from build123d import *

# Parameters (mm, degrees)
SKETCH1_W           = 5
SKETCH1_H           = 30
SKETCH1_R           = 1.55
BOSS_EXTRUDE1_DEPTH = 3
FILLET1_R           = 2.5


with BuildPart() as part:
    # Sketch1 → Boss-Extrude1 (new body)
    with BuildSketch(Plane(origin=(0, 0, 0), x_dir=(1, 0, 0), z_dir=(0, 1, 0))):
        Rectangle(SKETCH1_W, SKETCH1_H)
        with Locations(Location((0, 12, 0), (0, 0, 270))):
            Circle(SKETCH1_R, mode=Mode.SUBTRACT)
        with Locations(Location((0, -12, 0), (0, 0, 270))):
            Circle(SKETCH1_R, mode=Mode.SUBTRACT)
    extrude(amount=BOSS_EXTRUDE1_DEPTH)

    # Fillet1
    fillet1_edges = [part.edges().sort_by_distance(p)[0] for p in [
        (-2.5, 1.5, 15),
        (-2.5, 1.5, -15),
        (2.5, 1.5, -15),
        (2.5, 1.5, 15),
    ]]
    fillet(fillet1_edges, radius=FILLET1_R - 0.0001)  # a hair under: the kernel refuses the full size


solid = part.part
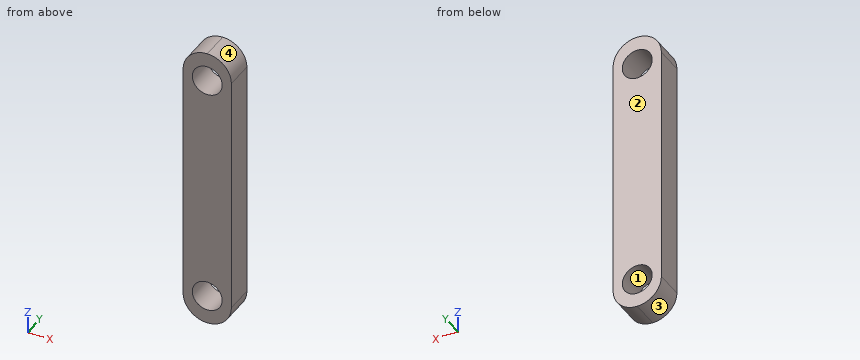
Build history of the part. All positions in model axes, mm. Face numbers are marked on the shaded views. Round coordinates to 2 decimals unless told otherwise and drop trailing zeros. Write each loop counter-clockwise with the first axis right and the second up, starting at its lowest first coordinate (ties: lowest second). Pieces come first, ordered by that corner, then holes. Notation, with made-up numbers: (62.5, -10) -> (121.5, -10) arc R10 cw to (121.5, 6) -> close; hole circle Ø11 at (78.25, 76). An arc over 180 degrees is marked (long way). Use one line per item in the form item = value.
Q1. Band-saw the part on A-A, the plane z = 12. Write the cut outline in (x, y).
Conclusion:
outline = (-2.5, 0) -> (-1.55, 0) -> (-1.55, 3) -> (-2.5, 3) -> close; (1.55, 0) -> (2.5, 0) -> (2.5, 3) -> (1.55, 3) -> close
Q2. Band-saw the part on B-B, the plane y = 2. State how many separate pieces and enclosed holes the cut face has, then the cut area to 3 significant figures.
Conclusion:
separate_pieces = 1
enclosed_holes = 2
area = 130 mm²
Q3. Drill centre lines: L1, parallel to Z at x = -0.6, y = 0.5; L2, parallel to Z at x = 1, y = 1.35; L3, parallel to X at y = 1.45, z = -12. Where is each one in solid material? Low to high.
Conclusion:
L1 = -14.93 to -13.43, -10.57 to 10.57, 13.43 to 14.93
L2 = -14.79 to -13.18, -10.82 to 10.82, 13.18 to 14.79
L3 = -2.5 to -1.55, 1.55 to 2.5
Q4. Band-saw the part on D-D, the plane x = 2.15. Write the cut outline in (y, z), then the cut area to 3 significant figures.
Conclusion:
outline = (0, -13.78) -> (3, -13.78) -> (3, 13.78) -> (0, 13.78) -> close
area = 82.7 mm²
Q5. Band-saw the part on C-C, the plane x = 0.75. Write the cut outline in (y, z).
Conclusion:
outline = (0, -14.88) -> (3, -14.88) -> (3, -13.36) -> (0, -13.36) -> close; (0, -10.64) -> (3, -10.64) -> (3, 10.64) -> (0, 10.64) -> close; (0, 13.36) -> (3, 13.36) -> (3, 14.88) -> (0, 14.88) -> close
Q6. Two-plate mould, pull along Z, no slides. Class the marked faces 1, 2, 3 and 4: released by +Z, released by -Z, zero draft, split by the parting line, or undercut.
Conclusion:
face_1 = undercut
face_2 = zero draft
face_3 = released by -Z
face_4 = released by +Z
Q7. Drop a flat-ended pin along its axis: P1, Ø1, axis at x = -1.5, y = 1, coming from the -Z side. Give the stop position or say it passes through.
Conclusion:
P1 = -14.79
